```python
from build123d import *

# Parameters (mm, degrees)
SKETCH_1_W               = 100
SKETCH_1_H               = 130
EXTRUDE_1_DEPTH          = 3
SKETCH_2_R               = 2.1
CUT_EXTRUDE_1_DEPTH      = 83.060952956
CUT_EXTRUDE_2_DEPTH      = 83.060952956
CUT_EXTRUDE_2_DEPTH_BACK = 83.060952956
SKETCH_3_R               = 1.25
CUT_EXTRUDE_3_DEPTH      = 83.060952956
CUT_EXTRUDE_3_DEPTH_BACK = 83.060952956
SKETCH_4_R               = 12.5
SKETCH_5_W               = 140
SKETCH_5_H               = 130
EXTRUDE_2_DEPTH          = 3
CUT_EXTRUDE_4_DEPTH      = 201.833264177
CUT_EXTRUDE_4_DEPTH_BACK = 201.833264177
SKETCH_6_R               = 2.1


with BuildPart() as part:
    # 草图1 → 凸台-拉伸1 (new body)
    with BuildSketch(Plane.XY):
        Rectangle(SKETCH_1_W, SKETCH_1_H)
    extrude(amount=EXTRUDE_1_DEPTH)

    # 草图2 → 切除-拉伸1 (cut, through all)
    with BuildSketch(Plane.XY.offset(3)):
        with Locations((-40, 55)):
            Circle(SKETCH_2_R)
        with Locations((-20, 55)):
            Circle(SKETCH_2_R)
        with Locations((0, 55)):
            Circle(SKETCH_2_R)
        with Locations((20, 55)):
            Circle(SKETCH_2_R)
        with Locations((40, 55)):
            Circle(SKETCH_2_R)
        with Locations((-40, 0)):
            Circle(SKETCH_2_R)
        with Locations((-40, -55)):
            Circle(SKETCH_2_R)
        with Locations((-40, -110)):
            Circle(SKETCH_2_R)
        with Locations((-40, -165)):
            Circle(SKETCH_2_R)
        with Locations((-40, -220)):
            Circle(SKETCH_2_R)
        with Locations((-40, -275)):
            Circle(SKETCH_2_R)
        with Locations((-40, -330)):
            Circle(SKETCH_2_R)
        with Locations((-40, -385)):
            Circle(SKETCH_2_R)
        with Locations((40, -385)):
            Circle(SKETCH_2_R)
        with Locations((40, -330)):
            Circle(SKETCH_2_R)
        with Locations((40, -275)):
            Circle(SKETCH_2_R)
        with Locations((40, -220)):
            Circle(SKETCH_2_R)
        with Locations((40, -165)):
            Circle(SKETCH_2_R)
        with Locations((40, -110)):
            Circle(SKETCH_2_R)
        with Locations(Location((40, -55, 0), (0, 0, 180))):
            Circle(SKETCH_2_R)
        with Locations(Location((40, 0, 0), (0, 0, 180))):
            Circle(SKETCH_2_R)
        with Locations(Location((20, -55, 0), (0, 0, 180))):
            Circle(SKETCH_2_R)
        with Locations(Location((0, -55, 0), (0, 0, 180))):
            Circle(SKETCH_2_R)
        with Locations(Location((-20, -55, 0), (0, 0, 180))):
            Circle(SKETCH_2_R)
    extrude(amount=-CUT_EXTRUDE_1_DEPTH, mode=Mode.SUBTRACT)

    # 草图3 → 切除-拉伸2 (cut, two sides: drawn at the far end of the back side and taken through both)
    with BuildSketch(Plane(origin=(0, 0, 0), x_dir=(-1, 0, 0), z_dir=(0, 0, -1)).offset(-CUT_EXTRUDE_2_DEPTH_BACK)):
        with Locations((19.042165039, -15)):
            Circle(SKETCH_3_R)
        with Locations((0.042165039, -34)):
            Circle(SKETCH_3_R)
        with Locations((-18.957834961, -15)):
            Circle(SKETCH_3_R)
        with Locations((0.042165039, 4)):
            Circle(SKETCH_3_R)
    extrude(amount=CUT_EXTRUDE_2_DEPTH + CUT_EXTRUDE_2_DEPTH_BACK, mode=Mode.SUBTRACT)

    # 草图4 → 切除-拉伸3 (cut, two sides: drawn at the far end of the back side and taken through both)
    with BuildSketch(Plane(origin=(0, 0, 0), x_dir=(-1, 0, 0), z_dir=(0, 0, -1)).offset(-CUT_EXTRUDE_3_DEPTH_BACK)):
        with Locations((0.042165039, -15)):
            Circle(SKETCH_4_R)
    extrude(amount=CUT_EXTRUDE_3_DEPTH + CUT_EXTRUDE_3_DEPTH_BACK, mode=Mode.SUBTRACT)

    # 草图5 → 凸台-拉伸2 (add)
    with BuildSketch(Plane.XY.offset(3)):
        with Locations((120, 0)):
            Rectangle(SKETCH_5_W, SKETCH_5_H)
    extrude(amount=-EXTRUDE_2_DEPTH)

    # 草图6 → 切除-拉伸4 (cut, two sides: drawn at the far end of the back side and taken through both)
    with BuildSketch(Plane.XY.offset(3).offset(-CUT_EXTRUDE_4_DEPTH_BACK)):
        with Locations((55, 55)):
            Circle(SKETCH_6_R)
        with Locations((70, 55)):
            Circle(SKETCH_6_R)
        with Locations((85, 55)):
            Circle(SKETCH_6_R)
        with Locations((100, 55)):
            Circle(SKETCH_6_R)
        with Locations((115, 55)):
            Circle(SKETCH_6_R)
        with Locations((130, 55)):
            Circle(SKETCH_6_R)
        with Locations((145, 55)):
            Circle(SKETCH_6_R)
        with Locations((145, -55)):
            Circle(SKETCH_6_R)
        with Locations((130, -55)):
            Circle(SKETCH_6_R)
        with Locations((115, -55)):
            Circle(SKETCH_6_R)
        with Locations((100, -55)):
            Circle(SKETCH_6_R)
        with Locations((85, -55)):
            Circle(SKETCH_6_R)
        with Locations((70, -55)):
            Circle(SKETCH_6_R)
        with Locations((55, -55)):
            Circle(SKETCH_6_R)
        with Locations((160, -55)):
            Circle(SKETCH_6_R)
        with Locations((175, -55)):
            Circle(SKETCH_6_R)
        with Locations((160, 55)):
            Circle(SKETCH_6_R)
        with Locations((175, 55)):
            Circle(SKETCH_6_R)
    extrude(amount=CUT_EXTRUDE_4_DEPTH + CUT_EXTRUDE_4_DEPTH_BACK, mode=Mode.SUBTRACT)


solid = part.part
```
For this review, take the finished solid that the model builds, in its own axes (mm). Round coordinates to 2 decimals unless told otherwise and drop trailing zeros.
(1) Clearance check with a flat-ended pin moving along its axis: P1, Ø3.5, axis at x = 40, y = 55, coming from the -Z side. State where the tip first meets the part, or that it passes through.
Returned:
P1: passes through
(2) We need section A-A (z = 1.2). State how many separate pieces and enclosed holes the cut face has, plus the area to 3 significant figures.
Returned:
separate pieces: 1
enclosed holes: 35
area: 30,300 mm2
(3) Wall thickness on line 1 along Y through (x, z) = (70, 2.3); line 2 along Y through (x, z) = (20, 0.7); line 3 along Y through (x, z) = (-20, 0.7): over which ranges is each line inside the solid? List them lowest first.
Returned:
line 1: y = -65 to -57.1, -52.9 to 52.9, 57.1 to 65
line 2: y = -65 to -57.1, -52.9 to -15.69, -14.31 to 52.9, 57.1 to 65
line 3: y = -65 to -57.1, -52.9 to -15.8, -14.2 to 52.9, 57.1 to 65
